The figure shows three views and two pictorial views of one solid part (mm, origin at its lowest corner). Answer the questions. Coordinates: 2 decimals unless noted, no trailing zeros. Order: outer loops, then holes, each group sorted by start corner. A loop starts at its lowest first (then second) coordinate and runs counter-clockwise, first axis right, second up. Notation, with made-up numbers: (-6, 11.25) -> (53, 11.25) arc R30 cw to (53, 47.25) -> close; hole circle Ø8 at (57.5, 59.25). An arc over 180 degrees is marked (long way). Return JSON: item names as keys, results as strings. Group by question number.
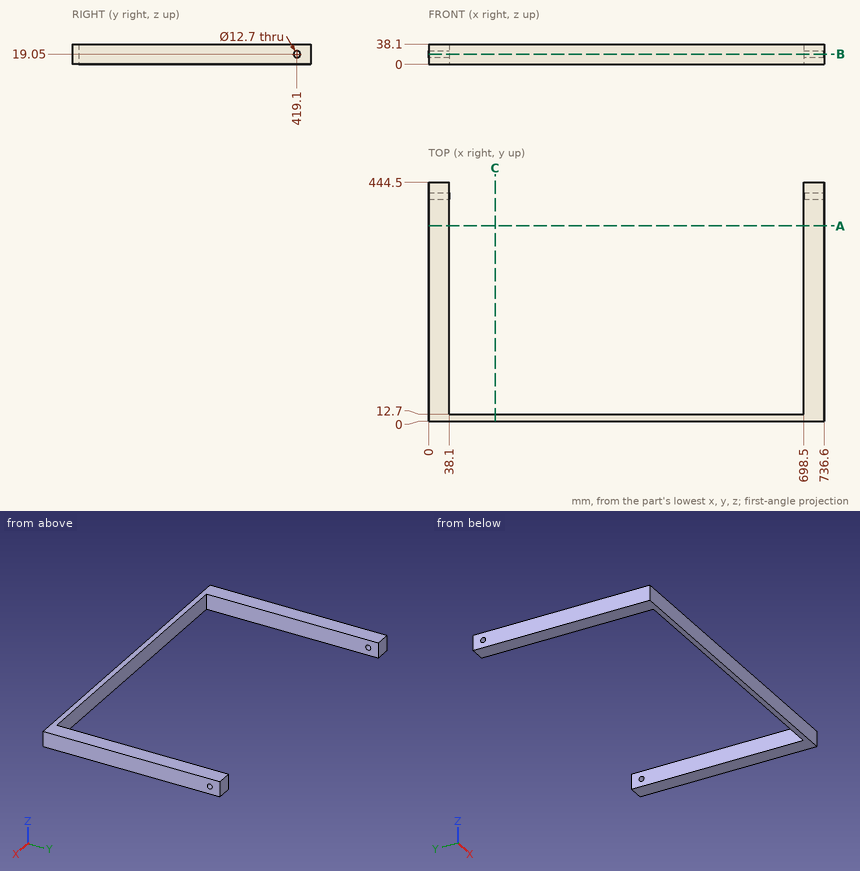
1. Find section C-C on x = 124. Determine the outline of the cut face in (y, z).
2. Given pin 1 (8 mm diameter, centred on x = 467, z = 24.5, fed in from +Y), flat-ended and moving along its own axis, determine where the tip first touches the part or whether it passes through.
3. Find section A-A on y = 363.5. Determine the outline of the cut face in (x, z).
4. Straight lines are drawn through the part: L1, parallel to X at y = 105, z = 3; L2, parallel to Y at x = 706, z = 19; L3, parallel to Z at x = 717, y = 419.1. For each, find the intervals that lie inside material, in ascending order.
5. Find section B-B on z = 19.05. Determine the outline of the cut face in (x, y), and give its area (3 significant figures).
Result:
{
 "1": {"outline": "(0, 0) -> (12.7, 0) -> (12.7, 38.1) -> (0, 38.1) -> close"},
 "2": {"pin 1": "y = 12.7"},
 "3": {"outline": "(0, 0) -> (38.1, 0) -> (38.1, 38.1) -> (0, 38.1) -> close; (698.5, 0) -> (736.6, 0) -> (736.6, 38.1) -> (698.5, 38.1) -> close"},
 "4": {"L1": "0 to 38.1, 698.5 to 736.6", "L2": "0 to 412.75, 425.45 to 444.5", "L3": "0 to 12.7, 25.4 to 38.1"},
 "5": {"outline": "(0, 0) -> (736.6, 0) -> (736.6, 412.75) -> (698.5, 412.75) -> (698.5, 12.7) -> (38.1, 12.7) -> (38.1, 412.75) -> (0, 412.75) -> close; (0, 425.45) -> (38.1, 425.45) -> (38.1, 444.5) -> (0, 444.5) -> close; (698.5, 425.45) -> (736.6, 425.45) -> (736.6, 444.5) -> (698.5, 444.5) -> close", "area": "41,300 mm^2"}
}
